from build123d import *

# Parameters (mm, degrees)
TAP_DRILL_FOR_M3X0_5_TAP1_D           = 2.5
TAP_DRILL_FOR_M3X0_5_TAP1_CSINK_D     = 2.55
TAP_DRILL_FOR_M3X0_5_TAP1_CSINK_ANGLE = 90
SKETCH5_R                             = 2.75
CUT_EXTRUDE1_DEPTH                    = 3
SKETCH6_R                             = 1.5
CUT_EXTRUDE2_DEPTH                    = 15.456832295


with BuildPart() as part:
    # Sketch1 → Revolve1 (revolve)
    with BuildSketch(Plane(origin=(0, 0, 0), x_dir=(0, 0, -1), z_dir=(1, 0, 0))):
        Polygon((0, 0), (-10, 0), (-10, -2), (-4.5, -2), (-4.5, -5), (0, -5), align=None)
    revolve(axis=Axis((0, 0, 0), (0, -1, 0)))

    # Tap Drill for M3x0.5 Tap1 (through all)
    with Locations(Plane(origin=(0, -2, 0), x_dir=(-1, 0, 0), z_dir=(0, -1, 0))):
        with Locations((4.949747468, 4.949747468), (-4.949747468, -4.949747468), (-4.949747468, 4.949747468), (4.949747468, -4.949747468)):
            CounterSinkHole(TAP_DRILL_FOR_M3X0_5_TAP1_D / 2, TAP_DRILL_FOR_M3X0_5_TAP1_CSINK_D / 2, counter_sink_angle=TAP_DRILL_FOR_M3X0_5_TAP1_CSINK_ANGLE)

    # Sketch5 → Cut-Extrude1 (cut)
    with BuildSketch(Plane(origin=(0, -5, 0), x_dir=(-1, 0, 0), z_dir=(0, -1, 0))):
        with Locations(Location((0, 0, 0), (0, 0, 90))):
            Circle(SKETCH5_R)
    extrude(amount=-CUT_EXTRUDE1_DEPTH, mode=Mode.SUBTRACT)

    # Sketch6 → Cut-Extrude2 (cut, through all)
    with BuildSketch(Plane(origin=(0, -2, 0), x_dir=(-1, 0, 0), z_dir=(0, -1, 0))):
        with Locations(Location((0, 0, 0), (0, 0, 90))):
            Circle(SKETCH6_R)
    extrude(amount=-CUT_EXTRUDE2_DEPTH, mode=Mode.SUBTRACT)


solid = part.part
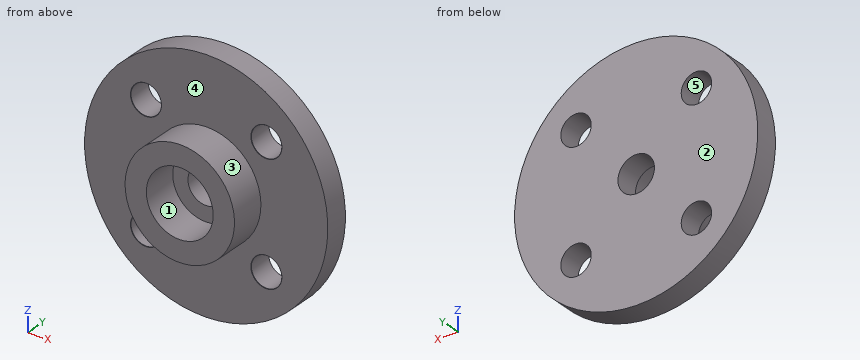
Build history of the part. All positions in model axes, mm. Face numbers are marked on the shaded views. A direction names the side the tool comes from. Round coordinates to 2 decimals unless told otherwise and drop trailing zeros. Write each loop counter-clockwise with the first axis right and the second up, starting at its lowest first coordinate (ties: lowest second). Pieces come first, ordered by that corner, then holes. Notation, with made-up numbers: (67, -1) - (113, -1) arc R18 cw to (113, 9) - close; hole circle Ø11 at (5, 23.5). An arc over 180 degrees is marked (long way). Use CSV: the item, a comma, the result in double quotes.
(1) Mould opens along X. For the marked faces 3, 4 and 5 say: pulls with the +X half, pulls with the -X half, needs draft (parallel to the pull), parting line crosses it, or undercut.
Response:
face 3,"parting line crosses it"
face 4,"needs draft"
face 5,"undercut"
(2) 3-axis set-ups, long thin cutter, end or side, ignore diameter. For the marked faces 1 and 2: which of +Z, -Z, +X, -X, +Y, -Y reach the whole face in a straight line?
Response:
face 1,"-Y"
face 2,"+Z, -Z, +X, -X, +Y"
(3) Pin check, flat tips, straight feed: P1, Ø1.5, axis at x = 4.95, z = -4.95, coming from the +Y side; P2, Ø4, axis at x = -4.95, z = -4.95, coming from the -Y side. Stop position of each tip, or through.
Response:
P1,"through"
P2,"y = -2"
(4) Wall check: line 1 (Y direction, x = 8, z = -4.5); line 2 (X direction, y = -2.15, z = 1.75); line 3 (X direction, y = -0.8, z = -0.75). Give the ranges that are in metal, low to high.
Response:
line 1,"-2 to 0"
line 2,"-4.15 to -2.12, 2.12 to 4.15"
line 3,"-9.97 to -1.3, 1.3 to 9.97"
(5) Band-saw the part on C-C (z = 3). Write the cut outline in (x, y), plus the area to 3 significant figures.
Response:
outline,"(-9.54, -2) - (-3.35, -2) - (-3.35, -5) - (3.35, -5) - (3.35, -2) - (9.54, -2) - (9.54, 0) - (-9.54, 0) - close"
area,"58.3 mm²"
(6) Band-saw the part on A-A (z = 0). Write the cut outline in (x, y).
Response:
outline,"(-10, -2) - (-4.5, -2) - (-4.5, -5) - (-2.75, -5) - (-2.75, -2) - (-1.5, -2) - (-1.5, 0) - (-10, 0) - close; (1.5, -2) - (2.75, -2) - (2.75, -5) - (4.5, -5) - (4.5, -2) - (10, -2) - (10, 0) - (1.5, 0) - close"
(7) Band-saw the part on D-D (y = -3.05). Write the cut outline in (x, z).
Response:
outline,"circle Ø9 at (0, 0); hole circle Ø5.5 at (0, 0)"
(8) Band-saw the part on B-B (x = 0). Write the cut outline in (y, z).
Response:
outline,"(-5, -4.5) - (-2, -4.5) - (-2, -10) - (0, -10) - (0, -1.5) - (-2, -1.5) - (-2, -2.75) - (-5, -2.75) - close; (-5, 2.75) - (-2, 2.75) - (-2, 1.5) - (0, 1.5) - (0, 10) - (-2, 10) - (-2, 4.5) - (-5, 4.5) - close"
